For this review, take the finished solid that the model builds, in its own axes (mm). Face numbers are marked on the shaded views. Round coordinates to 2 decimals unless told otherwise and drop trailing zeros. Loops run counter-clockwise (first coordinate to the right, second up) from the corner with the lowest first, then second, coordinate; pieces in that order, holes last.
1) Wall thickness on L1, parallel to X at y = 0, z = 33; L2, parallel to X at y = 0, z = 37; L3, parallel to Y at x = -16, z = 21: over which ranges is each line inside the solid? List them lowest first.
2) Take a section at A-A (y = 0). State the section outline as (x, z) points.
3) Mouldability with a two-part tool opening along X and no side actions: class the marked faces 1, 2 and 3 as pulls with the +X half, pulls with the -X half, needs draft (parallel to the pull), parting line crosses it, or undercut.
4) Take a section at B-B (x = 0). State the section outline as (y, z) points.
5) Take a section at D-D (y = -20). State the section outline as (x, z) points, then the cut area to 3 significant figures.
6) Insertion check: pin 1 (6 mm diameter, centred on x = -30, z = 20.5, fed in from -Y); pin 2 (14 mm diameter, centred on x = -19, z = 28.5, fed in from +Y). Each pin has a flat end and moves straight along its axis. Give the tip position at first contact, or say it passes through.
7) Take a section at C-C (z = 16.5). State the section outline as (x, y) points, then the cut area to 3 significant figures.
```python
from build123d import *

# Parameters (mm, degrees)
F0_W          = 83.8607475162
F0_H          = 64.1791447997
F1_DEPTH      = 48.26
F2_R          = 18.8345255186
F3_DEPTH      = 44.196
F3_DEPTH_BACK = 44.196
F4_R          = 12.5378078108
F5_DEPTH      = 44.197
F5_DEPTH_BACK = 44.197
F7_DEPTH      = 44.197
F7_DEPTH_BACK = 44.197
F8_R          = 6.1393043091
F8_R_2        = 6.139306213
F9_DEPTH      = 154
F9_DEPTH_BACK = 47.3427378962


# Not quite as in the source:
# - an extrude ends at something that could not be found from the text; its depth is read off the source's solid


with BuildPart() as f1:
    # F0 (on Top) → F1 (new body)
    with BuildSketch(Plane.XY):
        Rectangle(F0_W, F0_H)
    extrude(amount=F1_DEPTH)

    # F2 (on Front) → F3 (join, two sides)
    with BuildSketch(Plane.XZ) as f3_sk:
        with Locations((0, 47.7778092027)):
            Circle(F2_R)
    extrude(amount=F3_DEPTH)
    extrude(f3_sk.sketch, amount=-F3_DEPTH_BACK)

    # F4 (on Front) → F5 (cut, two sides)
    with BuildSketch(Plane.XZ) as f5_sk:
        with Locations((0, 48.2809320092)):
            Circle(F4_R)
    extrude(amount=-F5_DEPTH, mode=Mode.SUBTRACT)
    extrude(f5_sk.sketch, amount=F5_DEPTH_BACK, mode=Mode.SUBTRACT)

    # F6 (on Front) → F7 (cut, two sides)
    with BuildSketch(Plane.XZ) as f7_sk:
        Polygon((-43.335814029, 47.3417378962), (42.9494790733, 47.3417378962), (48.3834594488, 70.2134892344), (-43.335814029, 70.2134892344), align=None)
    extrude(amount=-F7_DEPTH, mode=Mode.SUBTRACT)
    extrude(f7_sk.sketch, amount=F7_DEPTH_BACK, mode=Mode.SUBTRACT)

    # F8 (on Top) → F9 (cut, two sides)
    with BuildSketch(Plane.XY) as f9_sk:
        with Locations((-30.2355084568, 0)):
            Circle(F8_R)
        with Locations((29.3797850609, 0)):
            Circle(F8_R_2)
    extrude(amount=-F9_DEPTH, mode=Mode.SUBTRACT)
    extrude(f9_sk.sketch, amount=F9_DEPTH_BACK, mode=Mode.SUBTRACT)


solid = f1.part
```
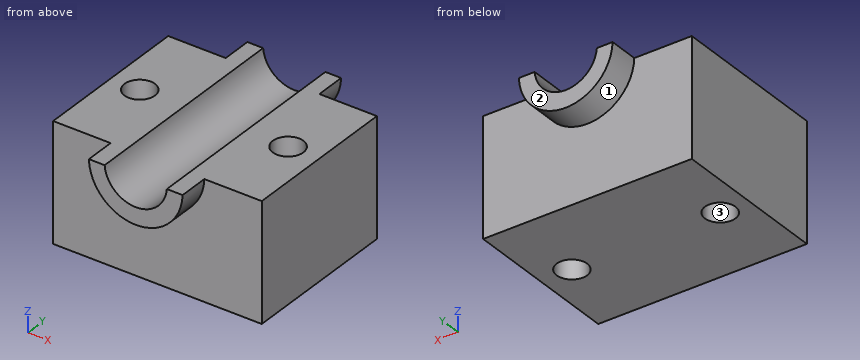
Response:
1. L1: x = -41.93 to -36.37, -24.1 to 23.24, 35.52 to 41.93
1. L2: x = -41.93 to -36.37, -24.1 to -5.47, 5.47 to 23.24, 35.52 to 41.93
1. L3: y = -32.09 to 32.09
2. outline: (-41.93, 0) - (-36.37, 0) - (-36.37, 47.34) - (-41.93, 47.34) - close; (-24.1, 0) - (23.24, 0) - (23.24, 47.34) - (12.5, 47.34) arc R12.54 cw to (-12.5, 47.34) - (-24.1, 47.34) - close; (35.52, 0) - (41.93, 0) - (41.93, 47.34) - (35.52, 47.34) - close
3. face 1: parting line crosses it
3. face 2: needs draft
3. face 3: undercut
4. outline: (-44.2, 28.94) - (-32.09, 28.94) - (-32.09, 0) - (32.09, 0) - (32.09, 28.94) - (44.2, 28.94) - (44.2, 35.74) - (-44.2, 35.74) - close
5. outline: (-41.93, 0) - (41.93, 0) - (41.93, 47.34) - (12.5, 47.34) arc R12.54 cw to (-12.5, 47.34) - (-41.93, 47.34) - close
5. area: 3,750 mm2
6. pin 1: stops at y = -32.09
6. pin 2: stops at y = 32.09
7. outline: (-41.93, -32.09) - (41.93, -32.09) - (41.93, 32.09) - (-41.93, 32.09) - close; hole circle Ø12.28 at (-30.24, 0); hole circle Ø12.28 at (29.38, 0)
7. area: 5,150 mm2
